Read the model definition and answer for the solid it produces. Units are mm, in the model's axes. A direction names the side the tool comes from. Coordinates: 2 decimals unless noted, no trailing zeros. Write each loop counter-clockwise with the first axis right and the second up, starting at its lowest first coordinate (ties: lowest second). Pieces come first, ordered by that corner, then holes. Notation, with made-up numbers: M 37,17.5 L 52,17.5 A17 cw 52,42.5 Z; hole C -15.75,3.25 d4. An arc over 180 degrees is marked long. Use a Markdown table: item, result. Add a question column.
from build123d import *

# Parameters (mm, degrees)
BOSS_EXTRUDE1_DEPTH = 5
SKETCH2_R           = 2.5
CUT_EXTRUDE1_DEPTH  = 59.523499554
SKETCH3_R           = 1
BOSS_EXTRUDE2_DEPTH = 7.5
CUT_EXTRUDE3_REACH  = 71.82
SKETCH5_W           = 5
SKETCH5_H           = 18
FILLET1_R           = 3
SKETCH6_R           = 2
BOSS_EXTRUDE3_DEPTH = 7.5
SKETCH7_W           = 5.3
SKETCH7_H           = 20
CUT_EXTRUDE4_DEPTH  = 10
FILLET2_R           = 3
CUT_EXTRUDE5_DEPTH  = 60.160797831
FILLET4_R           = 10
SKETCH10_R          = 2
BOSS_EXTRUDE4_DEPTH = 22.5
SKETCH11_W          = 15
SKETCH11_H          = 20
SKETCH11_W_2        = 5.3
CUT_EXTRUDE6_DEPTH  = 10
FILLET5_R           = 2


with BuildPart() as part:
    # Sketch1 → Boss-Extrude1 (new body)
    with BuildSketch(Plane.XY):
        with BuildLine():
            Line((28.94427191, 4.472135955), (8.94427191, 44.472135955))
            ThreePointArc((8.94427191, 44.472135955), (0, 50), (-8.94427191, 44.472135955))
            Line((-8.94427191, 44.472135955), (-28.94427191, 4.472135955))
            ThreePointArc((-28.94427191, 4.472135955), (-29.827586533, 1.848930213), (-29.957965225, -0.915930449))
            Line((-29.957965225, -0.915930449), (-28.878099151, -12.656198302))
            ThreePointArc((-28.878099151, -12.656198302), (0, -39), (28.878099151, -12.656198302))
            Line((28.878099151, -12.656198302), (29.957965225, -0.915930449))
            ThreePointArc((29.957965225, -0.915930449), (29.827586533, 1.848930213), (28.94427191, 4.472135955))
        make_face()
    extrude(amount=BOSS_EXTRUDE1_DEPTH)

    # Sketch2 → Cut-Extrude1 (cut, through all)
    with BuildSketch(Plane.XY.offset(5)):
        with Locations((0, 40)):
            Circle(SKETCH2_R)
        with Locations((22.5, 0)):
            Circle(SKETCH2_R)
        with Locations((-22.5, 0)):
            Circle(SKETCH2_R)
    extrude(amount=-CUT_EXTRUDE1_DEPTH, mode=Mode.SUBTRACT)

    # Sketch3 → Boss-Extrude2 (add, symmetric)
    with BuildSketch(Plane(origin=(0, 0, 0), x_dir=(0, 0, -1), z_dir=(1, 0, 0))):
        with BuildLine():
            Line((-5, 22.472135955), (-5, 14.472135955))
            Line((-5, 14.472135955), (-10, 14.472135955))
            ThreePointArc((-10, 14.472135955), (-14, 18.472135955), (-10, 22.472135955))
            Line((-10, 22.472135955), (-5, 22.472135955))
        make_face()
        with Locations((-10, 18.472135955)):
            Circle(SKETCH3_R, mode=Mode.SUBTRACT)
    extrude(amount=BOSS_EXTRUDE2_DEPTH, both=True)

    # Cut-Extrude3: up to this face of the body (flat: up to its plane)
    cut_extrude3_end = Plane(part.part.faces().sort_by_distance((0, 14.472135955, 7.5))[0])
    # Sketch5 → Cut-Extrude3 (cut, up to the picked face)
    with BuildSketch(Plane(origin=(0, 22.472135955, 0), x_dir=(1, 0, 0), z_dir=(0, 1, 0)), mode=Mode.PRIVATE) as cut_extrude3_sk1:
        with Locations((0, -14)):
            Rectangle(SKETCH5_W, SKETCH5_H)
    cut_extrude3_tool1 = split(extrude(cut_extrude3_sk1.sketch, amount=-CUT_EXTRUDE3_REACH, mode=Mode.PRIVATE), bisect_by=cut_extrude3_end, keep=Keep.BOTH, mode=Mode.PRIVATE)
    add(cut_extrude3_tool1.solids().sort_by(Axis((0, 22.472136, 14), (0, -1, 0)))[0], mode=Mode.SUBTRACT)

    # Fillet1
    fillet1_edges = [part.edges().sort_by_distance(p)[0] for p in [
        (5, 22.472135955, 5),
        (5, 14.472135955, 5),
        (-5, 14.472135955, 5),
        (-5, 22.472135955, 5),
    ]]
    fillet(fillet1_edges, radius=FILLET1_R)

    # Sketch6 → Boss-Extrude3 (add, symmetric)
    with BuildSketch(Plane(origin=(0, 0, 0), x_dir=(0, 0, -1), z_dir=(1, 0, 0))):
        with BuildLine():
            Line((-5, 26.472135955), (-5, 36.472135955))
            Line((-5, 36.472135955), (-10, 36.472135955))
            ThreePointArc((-10, 36.472135955), (-15, 31.472135955), (-10, 26.472135955))
            Line((-10, 26.472135955), (-5, 26.472135955))
        make_face()
        with Locations((-10, 31.472135955)):
            Circle(SKETCH6_R, mode=Mode.SUBTRACT)
    extrude(amount=BOSS_EXTRUDE3_DEPTH, both=True)

    # Sketch7 → Cut-Extrude4 (cut)
    with BuildSketch(Plane(origin=(0, 36.472135955, 0), x_dir=(1, 0, 0), z_dir=(0, 1, 0))):
        with Locations((0, -15)):
            Rectangle(SKETCH7_W, SKETCH7_H)
    extrude(amount=-CUT_EXTRUDE4_DEPTH, mode=Mode.SUBTRACT)

    # Fillet2
    # the kernel refuses this fillet: 3 mm, written as the material it adds along each edge
    with BuildSketch(Plane(origin=(7.5, 26.472135955, 5), x_dir=(0, -1, 0), z_dir=(-1, 0, 0)), Plane(origin=(2.65, 36.472135955, 5), x_dir=(0, 1, 0), z_dir=(1, 0, 0)), Plane(origin=(-7.5, 36.472135955, 5), x_dir=(0, 1, 0), z_dir=(1, 0, 0)), Plane(origin=(-2.65, 26.472135955, 5), x_dir=(0, -1, 0), z_dir=(-1, 0, 0))) as fillet2_piece_1:
        with BuildLine():
            CenterArc((FILLET2_R, FILLET2_R), FILLET2_R, 180, 90)
            Line((0, FILLET2_R), (0, 0))
            Line((0, 0), (FILLET2_R, 0))
        make_face()
    extrude(amount=4.85)
    with BuildSketch(Plane(origin=(7.5, 26.472135955, 5), x_dir=(0, -1, 0), z_dir=(-1, 0, 0))) as fillet2_piece_2_section:
        with BuildLine():
            CenterArc((FILLET2_R, FILLET2_R), FILLET2_R, 180, 90)
            Line((0, FILLET2_R), (0, 0))
            Line((0, 0), (FILLET2_R, 0))
        make_face()
    fillet2_piece_2 = extrude(amount=12.35, mode=Mode.PRIVATE)
    fillet2_piece_2 = split(fillet2_piece_2, bisect_by=Plane(origin=(-2.65, 25.792950612, 5.679185343), z_dir=(-1, 0, 0)), keep=Keep.TOP, mode=Mode.PRIVATE)
    add(fillet2_piece_2)
    with BuildSketch(Plane(origin=(-4.85, 36.472135955, 5), x_dir=(0, 1, 0), z_dir=(1, 0, 0))) as fillet2_piece_3_section:
        with BuildLine():
            CenterArc((FILLET2_R, FILLET2_R), FILLET2_R, 180, 90)
            Line((0, FILLET2_R), (0, 0))
            Line((0, 0), (FILLET2_R, 0))
        make_face()
    fillet2_piece_3 = extrude(amount=12.35, mode=Mode.PRIVATE)
    fillet2_piece_3 = split(fillet2_piece_3, bisect_by=Plane(origin=(-2.65, 37.151321298, 5.679185343), z_dir=(-1, 0, 0)), keep=Keep.TOP, mode=Mode.PRIVATE)
    add(fillet2_piece_3)
    with BuildSketch(Plane(origin=(-7.5, 36.472135955, 5), x_dir=(0, 1, 0), z_dir=(1, 0, 0))) as fillet2_piece_4_section:
        with BuildLine():
            CenterArc((FILLET2_R, FILLET2_R), FILLET2_R, 180, 90)
            Line((0, FILLET2_R), (0, 0))
            Line((0, 0), (FILLET2_R, 0))
        make_face()
    fillet2_piece_4 = extrude(amount=12.35, mode=Mode.PRIVATE)
    fillet2_piece_4 = split(fillet2_piece_4, bisect_by=Plane(origin=(2.65, 37.151321298, 5.679185343), z_dir=(1, 0, 0)), keep=Keep.TOP, mode=Mode.PRIVATE)
    add(fillet2_piece_4)
    with BuildSketch(Plane(origin=(4.85, 26.472135955, 5), x_dir=(0, -1, 0), z_dir=(-1, 0, 0))) as fillet2_piece_5_section:
        with BuildLine():
            CenterArc((FILLET2_R, FILLET2_R), FILLET2_R, 180, 90)
            Line((0, FILLET2_R), (0, 0))
            Line((0, 0), (FILLET2_R, 0))
        make_face()
    fillet2_piece_5 = extrude(amount=12.35, mode=Mode.PRIVATE)
    fillet2_piece_5 = split(fillet2_piece_5, bisect_by=Plane(origin=(2.65, 25.792950612, 5.679185343), z_dir=(1, 0, 0)), keep=Keep.TOP, mode=Mode.PRIVATE)
    add(fillet2_piece_5)

    # Sketch8 → Cut-Extrude5 (cut, through all)
    with BuildSketch(Plane.XY.offset(5)):
        with BuildLine():
            Line((-25.922962794, -23), (25.922962794, -23))
            ThreePointArc((25.922962794, -23), (0, -39), (-25.922962794, -23))
        make_face()
    extrude(amount=-CUT_EXTRUDE5_DEPTH, mode=Mode.SUBTRACT)

    # Fillet4
    fillet4_edges = [part.edges().sort_by_distance(p)[0] for p in [
        (25.922962794, -23, 2.5),
        (-25.922962794, -23, 2.5),
    ]]
    fillet(fillet4_edges, radius=FILLET4_R)

    # Sketch10 → Boss-Extrude4 (add, symmetric)
    with BuildSketch(Plane(origin=(0, 0, 0), x_dir=(0, 0, -1), z_dir=(1, 0, 0))):
        with BuildLine():
            Line((-5, -17), (-10, -17))
            ThreePointArc((-10, -17), (-15, -12), (-10, -7))
            Line((-10, -7), (-5, -7))
            Line((-5, -7), (-5, -17))
        make_face()
        with Locations(Location((-10, -12, 0), (0, 0, 180))):
            Circle(SKETCH10_R, mode=Mode.SUBTRACT)
    extrude(amount=BOSS_EXTRUDE4_DEPTH, both=True)

    # Sketch11 → Cut-Extrude6 (cut)
    with BuildSketch(Plane.XZ.offset(17)):
        with Locations((0, 15)):
            Rectangle(SKETCH11_W, SKETCH11_H)
        with Locations((-15, 15)):
            Rectangle(SKETCH11_W_2, SKETCH11_H)
    cut_extrude6 = extrude(amount=-CUT_EXTRUDE6_DEPTH, mode=Mode.SUBTRACT)

    # Mirror1: Cut-Extrude6 across plane
    add(cut_extrude6.mirror(Plane(origin=(0, 0, 0), x_dir=(0, 0, 1), z_dir=(1, 0, 0))), mode=Mode.SUBTRACT)

    # Fillet5
    fillet5_edges = [part.edges().sort_by_distance(p)[0] for p in [
        (20.075, -17, 5),
        (20.075, -7, 5),
        (-9.925, -17, 5),
        (-20.075, -17, 5),
        (-9.925, -7, 5),
        (-20.075, -7, 5),
        (9.925, -7, 5),
        (9.925, -17, 5),
    ]]
    fillet(fillet5_edges, radius=FILLET5_R)


solid = part.part
Item 1: Determine the mould class of faces 1 (the cylindrical face through (-10, -14, 10)), 2 (the cylindrical face through (-5, 23, 6.3)), 3 (the cylindrical face through (29.835, 1.811, 2.465)), 4 (the cylindrical face through (-5.035, 19.464, 10.13)) for opening direction Z: pulls with the +Z half, pulls with the -Z half, needs draft (parallel to the pull), parting line crosses it, or undercut.
Item 2: Find section B-B on y = 0. Give the vertices of the cut face in (x, z), then the cut area to 3 significant figures.
Item 3: Find section C-C on z = 2.75. Give the vertices of the cut face in (x, y), then the cut area to 3 significant figures.
Item 4: Consider probe 1 along Y at (x, z) = (-5.55, 10); probe 2 along X at (y, z) = (-14.5, 8); probe 3 along Z at (x, y) = (20, -12). Determine where each line is inside the solid, lowest interval first.
Item 5: Each of these flat-tipped pins is pushed along its axis until it touches: pin 1 (8 mm diameter, centred on x = -20, z = 13, fed in from +Y); pin 2 (12 mm diameter, centred on x = 1, y = -10, fed in from +Z); pin 3 (1.6 mm diameter, centred on x = 5.5, z = 9, fed in from +Y). Where does it stop, or does it pass through?
Item 6: Find section D-D on x = 6.5. Give the vertices of the cut face in (y, z), then the cut area to 3 significant figures.
Item 7: For faces 5 (the cylindrical face through (20, 0, 3)), 6 (the flat face through (0, 6, 0)), 7 (the flat face through (-20, -17, 8)), 8 (the flat face through (7.5, -12.1, 7.7)), 9 (the flat face through (-5, 26.472, 9)), determine the directions among +Z, -Z, +X, -X, +Y, -Y from which every point of the face is accessible in a straight line to the end or side of a thin tool.
Item 8: Find section A-A on x = 0. Give the vertices of the cut face in (y, z), then the cut area to 3 significant figures.
Geometry says:
| question | item | result |
|---|---|---|
| 1 | face 1 | undercut |
| 1 | face 2 | pulls with the +Z half |
| 1 | face 3 | needs draft |
| 1 | face 4 | undercut |
| 2 | outline | M -30,0 L -25,0 L -25,5 L -30,5 Z; M -20,0 L 20,0 L 20,5 L -20,5 Z; M 25,0 L 30,0 L 30,5 L 25,5 Z |
| 2 | area | 250 mm2 |
| 3 | outline | M -29.96,-0.92 L -28.88,-12.66 A29 ccw -28.64,-14.58 A10 ccw -18.76,-23 L 18.76,-23 A10 ccw 28.64,-14.58 A29 ccw 28.88,-12.66 L 29.96,-0.92 A10 ccw 28.94,4.47 L 8.94,44.47 A10 ccw -8.94,44.47 L -28.94,4.47 A10 ccw Z; hole C -22.5,0 d5; hole C 0,40 d5; hole C 22.5,0 d5 |
| 3 | area | 3,090 mm2 |
| 4 | probe 1 | y = 14.47 to 17.47, 19.47 to 22.47, 26.47 to 29.47, 33.47 to 36.47 |
| 4 | probe 2 | x = -22.5 to -17.65, -12.35 to -7.5, 7.5 to 12.35, 17.65 to 22.5 |
| 4 | probe 3 | z = 0 to 8, 12 to 15 |
| 5 | pin 1 | stops at y = -7 |
| 5 | pin 2 | stops at z = 5 |
| 5 | pin 3 | stops at y = 36.47 |
| 6 | outline | M -23,0 L 47.6,0 L 47.6,5 L 39.47,5 A3 cw 36.47,8 L 36.47,10 A5 ccw 26.47,10 L 26.47,8 A3 cw 24.47,5.17 A3 cw 22.47,8 L 22.47,10 A4 ccw 14.47,10 L 14.47,8 A3 cw 11.47,5 L -23,5 Z; hole C 18.47,10 d2; hole C 31.47,10 d4 |
| 6 | area | 499 mm2 |
| 7 | face 5 | +Z, -Z |
| 7 | face 6 | -Z, +X, -X, +Y, -Y |
| 7 | face 7 | +Z, +X, -X, -Y |
| 7 | face 8 | +Z, -Y |
| 7 | face 9 | +Z, +X, -X |
| 8 | outline | M -23,0 L 37.5,0 L 37.5,5 L -23,5 Z; M 42.5,0 L 50,0 L 50,5 L 42.5,5 Z |
| 8 | area | 340 mm2 |
